Here's how the part is built. I have some questions about the finished solid (model axes, mm). Coordinates: 2 decimals unless noted, no trailing zeros. Answer in a Markdown table with one row per item. Add a question column.
Item 1: If I drill on line 1 along Y through (x, z) = (165.85, 1.8); line 2 along Y through (x, z) = (270, 1.5); line 3 along Y through (x, z) = (45, 2.4), over which ranges is the centre line in solid material (lowest first)? Write a range as from..to.
Item 2: I want a section at A-A (z = 2.3). Count the separate pieces of the cut face and the enclosed holes in it, plus the area to 3 significant figures.
Item 3: Thinking about a two-plate mould opening in Y: for faces 1 (the cylindrical face through (305.709, 158.724, 1.521)), 2 (the flat face through (320.07, 166.18, 1.52)), 3 (the flat face through (163, 91, 3)), which applies, +Y half, -Y half, draft (parallel to the pull), parting line (faces both ways), or undercut?
```python
from build123d import *

# Parameters (mm, degrees)
SKETCH_1_W          = 330
SKETCH_1_H          = 180
EXTRUDE_1_DEPTH     = 3
SKETCH_2_R          = 1.6
CUT_EXTRUDE_1_DEPTH = 376.910893697
SKETCH_3_R          = 1.6
CUT_EXTRUDE_2_DEPTH = 376.910893697
CUT_EXTRUDE_3_REACH = 377.911
SKETCH_4_W          = 100
SKETCH_4_H          = 5
CUT_EXTRUDE_4_REACH = 377.911


with BuildPart() as part:
    # 草图1 → 凸台-拉伸1 (new body)
    with BuildSketch(Plane.XY):
        with Locations((165, 90)):
            Rectangle(SKETCH_1_W, SKETCH_1_H)
    extrude(amount=EXTRUDE_1_DEPTH)

    # 草图2 → 切除-拉伸1 (cut, through all)
    with BuildSketch(Plane.XY.offset(3)):
        with Locations((33.77, 166.83)):
            Circle(SKETCH_2_R)
        with Locations((165.85, 166.83)):
            Circle(SKETCH_2_R)
        with Locations((10.91, 9.35)):
            Circle(SKETCH_2_R)
        with Locations((165.85, 9.35)):
            Circle(SKETCH_2_R)
    extrude(amount=-CUT_EXTRUDE_1_DEPTH, mode=Mode.SUBTRACT)

    # 草图3 → 切除-拉伸2 (cut, through all)
    with BuildSketch(Plane.XY.offset(3)):
        with Locations((3, 160)):
            Circle(SKETCH_3_R)
        with Locations((3, 140)):
            Circle(SKETCH_3_R)
        with Locations((3, 45)):
            Circle(SKETCH_3_R)
        with Locations((3, 25)):
            Circle(SKETCH_3_R)
        with Locations((15, 3)):
            Circle(SKETCH_3_R)
        with Locations((35, 3)):
            Circle(SKETCH_3_R)
        with Locations((155, 3)):
            Circle(SKETCH_3_R)
        with Locations((175, 3)):
            Circle(SKETCH_3_R)
        with Locations((25, 176)):
            Circle(SKETCH_3_R)
        with Locations((45, 176)):
            Circle(SKETCH_3_R)
        with Locations((270, 176)):
            Circle(SKETCH_3_R)
        with Locations((290, 176)):
            Circle(SKETCH_3_R)
        with Locations((270, 3)):
            Circle(SKETCH_3_R)
        with Locations((290, 3)):
            Circle(SKETCH_3_R)
        with Locations((327, 5)):
            Circle(SKETCH_3_R)
        with Locations((327, 175)):
            Circle(SKETCH_3_R)
    extrude(amount=-CUT_EXTRUDE_2_DEPTH, mode=Mode.SUBTRACT)

    # 草图4 → 切除-拉伸3 (cut, up to next)
    with BuildSketch(Plane.XY.offset(3), mode=Mode.PRIVATE) as cut_extrude_3_sk1:
        with Locations((90, 2.5)):
            Rectangle(SKETCH_4_W, SKETCH_4_H)
    cut_extrude_3_tool1 = extrude(cut_extrude_3_sk1.sketch, amount=-CUT_EXTRUDE_3_REACH, mode=Mode.PRIVATE) & part.part
    add(cut_extrude_3_tool1.solids().sort_by_distance((90, 2.5, 3))[0], mode=Mode.SUBTRACT)

    # 草图6 → 切除-拉伸4 (cut, up to next)
    with BuildSketch(Plane.XY.offset(3), mode=Mode.PRIVATE) as cut_extrude_4_sk1:
        with BuildLine():
            Line((330, 170), (330, 105))
            Line((330, 105), (309, 105))
            ThreePointArc((309, 105), (305.464466094, 106.464466094), (304, 110))
            Line((304, 110), (304, 153.132009018))
            ThreePointArc((304, 153.132009018), (305.75688445, 158.793373344), (310.410209207, 162.46546508))
            Line((310.410209207, 162.46546508), (330, 170))
        make_face()
    cut_extrude_4_tool1 = extrude(cut_extrude_4_sk1.sketch, amount=-CUT_EXTRUDE_4_REACH, mode=Mode.PRIVATE) & part.part
    add(cut_extrude_4_tool1.solids().sort_by_distance((317.469531, 135.038029, 3))[0], mode=Mode.SUBTRACT)


solid = part.part
```
Values follow:
| question | item | result |
|---|---|---|
| 1 | line 1 | y = 0..7.75, 10.95..165.23, 168.43..180 |
| 1 | line 2 | y = 0..1.4, 4.6..174.4, 177.6..180 |
| 1 | line 3 | y = 5..174.4, 177.6..180 |
| 2 | separate pieces | 1 |
| 2 | enclosed holes | 20 |
| 2 | area | 57,200 mm^2 |
| 3 | face 1 | undercut |
| 3 | face 2 | undercut |
| 3 | face 3 | draft |
